The model under review builds one solid part; all positions refer to its coordinate system, in mm. A direction names the side the tool comes from. Give positions to 0.01 mm unless a question says otherwise; leave off trailing zeros. Order: outer loops, then holes, each group sorted by start corner. A loop starts at its lowest first (then second) coordinate and runs counter-clockwise, first axis right, second up. Notation, with made-up numbers: (77, 1) - (83, 1) arc R29 ccw to (83, 29) - close; hole circle Ø11 at (84.25, 47). An arc over 180 degrees is marked (long way). Put each result on its own line as item: value.
```python
from build123d import *

# Parameters (mm, degrees)
F1_R     = 9.5
F1_R_2   = 5.5
F2_DEPTH = 7
F3_DEPTH = 12


# Not quite as in the source:
# - a feature of the source that left no trace in its solid (it failed there, or was rolled back) is left out


with BuildPart() as f2:
    # F1 (on Top) → F2 (new body)
    with BuildSketch(Plane.XY):
        Polygon((-6.0621778265, 43.1666666667), (-40.4145188433, -16.3333333333), (-34.3523410168, -26.8333333333), (34.3523410168, -26.8333333333), (40.4145188433, -16.3333333333), (6.0621778265, 43.1666666667), align=None)
        with Locations((-20.4959345562, -11.8333333333)):
            Circle(F1_R, mode=Mode.SUBTRACT)
        with Locations((20.4959345562, -11.8333333333)):
            Circle(F1_R, mode=Mode.SUBTRACT)
        Circle(F1_R, mode=Mode.SUBTRACT)
        with Locations((0, 23.6666666667)):
            Circle(F1_R, mode=Mode.SUBTRACT)
        with Locations((0, 23.6666666667)):
            Circle(F1_R)
        with Locations((0, 23.6666666667)):
            Circle(F1_R_2, mode=Mode.SUBTRACT)
        with Locations((-20.4959345562, -11.8333333333)):
            Circle(F1_R)
        with Locations((-20.4959345562, -11.8333333333)):
            Circle(F1_R_2, mode=Mode.SUBTRACT)
        Circle(F1_R)
        Circle(F1_R_2, mode=Mode.SUBTRACT)
        with Locations((20.4959345562, -11.8333333333)):
            Circle(F1_R)
        with Locations((20.4959345562, -11.8333333333)):
            Circle(F1_R_2, mode=Mode.SUBTRACT)
    extrude(amount=F2_DEPTH)

    # F1 (on Top) → F3 (join)
    with BuildSketch(Plane.XY):
        Polygon((-6.0621778265, 43.1666666667), (-40.4145188433, -16.3333333333), (-34.3523410168, -26.8333333333), (34.3523410168, -26.8333333333), (40.4145188433, -16.3333333333), (6.0621778265, 43.1666666667), align=None)
        with Locations((-20.4959345562, -11.8333333333)):
            Circle(F1_R, mode=Mode.SUBTRACT)
        with Locations((20.4959345562, -11.8333333333)):
            Circle(F1_R, mode=Mode.SUBTRACT)
        Circle(F1_R, mode=Mode.SUBTRACT)
        with Locations((0, 23.6666666667)):
            Circle(F1_R, mode=Mode.SUBTRACT)
    extrude(amount=F3_DEPTH)


solid = f2.part
```
(1) Take a section at D-D, the plane z = 9.5. Write out the cut boundary in (x, y), then the cut area to 3 significant figures.
The answers:
outline: (-40.41, -16.33) - (-34.35, -26.83) - (34.35, -26.83) - (40.41, -16.33) - (6.06, 43.17) - (-6.06, 43.17) - close; hole circle Ø19 at (-20.5, -11.83); hole circle Ø19 at (0, 0); hole circle Ø19 at (0, 23.67); hole circle Ø19 at (20.5, -11.83)
area: 2,420 mm^2
(2) Take a section at C-C, the plane x = 19.5. Write out the cut boundary in (y, z), then the cut area to 3 significant figures.
The answers:
outline: (-26.83, 0) - (-17.24, 0) - (-17.24, 7) - (-21.28, 7) - (-21.28, 12) - (-26.83, 12) - close; (-6.42, 0) - (19.89, 0) - (19.89, 12) - (-2.39, 12) - (-2.39, 7) - (-6.42, 7) - close
area: 390 mm^2
(3) Take a section at B-B, the plane y = 1.5. Write out the cut boundary in (x, z).
The answers:
outline: (-30.12, 0) - (-5.29, 0) - (-5.29, 7) - (-9.38, 7) - (-9.38, 12) - (-30.12, 12) - close; (5.29, 0) - (30.12, 0) - (30.12, 12) - (9.38, 12) - (9.38, 7) - (5.29, 7) - close
(4) For faces 1 (the flat face through (4.1, 19.6, 7)), 2 (the cylindrical face through (-1.19, -5.37, 3.45)), list the 3-axis set-ups (+Z, -Z, +X, -X, +Y, -Y) from which the entire face can be reached by the end or side of a thin tool; tool diameter is ignored.
The answers:
face 1: +Z
face 2: +Z, -Z
(5) Wall thickness on L1, parallel to Y at x = 0, z = 8.6; L2, parallel to X at y = -16, z = 4.25; L3, parallel to Y at x = 21, z = 8: over which ranges is each line inside the solid? List them lowest first.
The answers:
L1: -26.83 to -9.5, 9.5 to 14.17, 33.17 to 43.17
L2: -40.22 to -24.09, -16.91 to 16.91, 24.09 to 40.22
L3: -26.83 to -21.32, -2.35 to 17.29
(6) The part is to be moulded in two halves that separate along X. For faces 3 (the flat face through (-37.426, -21.51, 5.916)), 4 (the cylindrical face through (4.38, -8.43, 9.46)), 5 (the flat face through (0, 43.167, 6)), say which applies: pulls with the +X half, pulls with the -X half, needs draft (parallel to the pull), parting line crosses it, or undercut.
The answers:
face 3: pulls with the -X half
face 4: undercut
face 5: needs draft
(7) Take a section at A-A, the plane x = 0. Write out the cut boundary in (y, z), then the cut area to 3 significant figures.
The answers:
outline: (-26.83, 0) - (-5.5, 0) - (-5.5, 7) - (-9.5, 7) - (-9.5, 12) - (-26.83, 12) - close; (5.5, 0) - (18.17, 0) - (18.17, 7) - (14.17, 7) - (14.17, 12) - (9.5, 12) - (9.5, 7) - (5.5, 7) - close; (29.17, 0) - (43.17, 0) - (43.17, 12) - (33.17, 12) - (33.17, 7) - (29.17, 7) - close
area: 496 mm^2
(8) Clearance check with flat-ended pins moving along their axes: pin 1 Ø10 at (x, y) = (0, 0) entering from -Z; pin 2 Ø17.5 at (x, y) = (20.5, -11.83) entering from +Z; pin 3 Ø6 at (x, z) = (-21.5, 5.5) entering from +Y. State where each tip first meets the part, or that it passes through.
The answers:
pin 1: through
pin 2: z = 7
pin 3: y = 21.62
